Source: three-view drawing plus pictorial views. Frame: mm from the lowest corner of the part. A direction names the side the tool comes from. Give positions to 0.01 mm unless a question says otherwise; leave off trailing zeros. Write each loop counter-clockwise with the first axis right and the second up, starting at its lowest first coordinate (ties: lowest second). Pieces come first, ordered by that corner, then holes. Notation, with made-up numbers: M -14,-5.75 L 14,-5.75 A18 ccw 14,15.25 Z; hole C 57,82 d5. An arc over 180 degrees is marked long. Return JSON: item names as keys, results as strings.
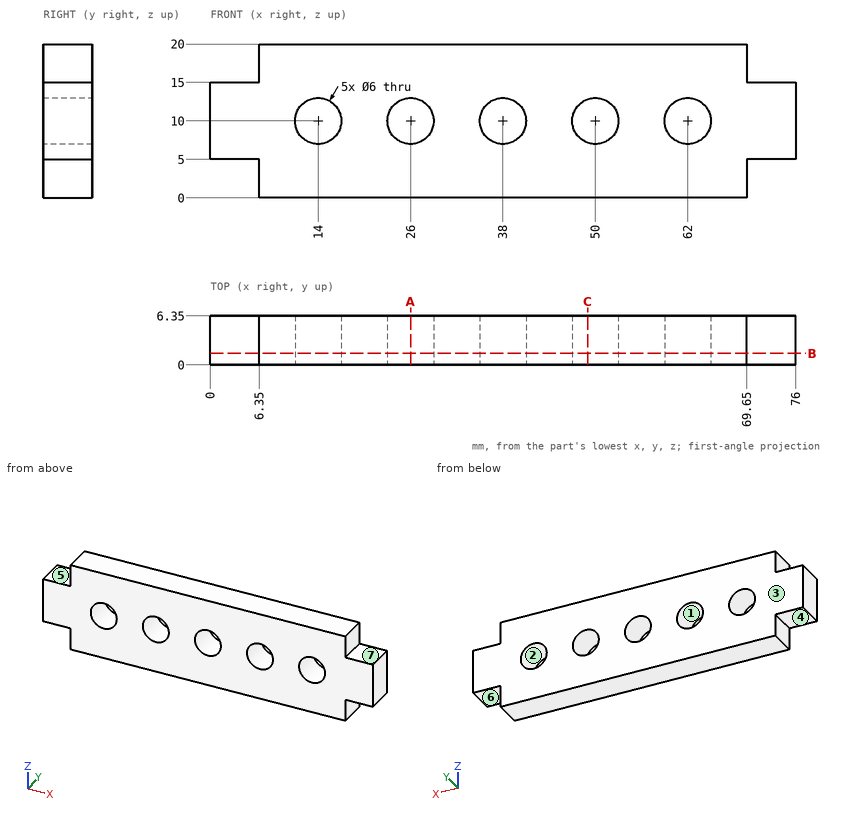
1) Line query: line 1 (X direction, y = 4, z = 10); line 2 (X direction, y = 3, z = 18); line 3 (Z direction, x = 51, y = 6). Output: solid intervals per line, ascending. Write a range as [from, to].
Numbers:
{"line 1": "x = [0, 11], [17, 23], [29, 35], [41, 47], [53, 59], [65, 76]", "line 2": "x = [6.35, 69.65]", "line 3": "z = [0, 7.17], [12.83, 20]"}
2) Cut plane A-A, the plane x = 26. Return the cut outline in (y, z), then the cut area to 3 significant figures.
Numbers:
{"outline": "M 0,0 L 6.35,0 L 6.35,7 L 0,7 Z; M 0,13 L 6.35,13 L 6.35,20 L 0,20 Z", "area": "88.9 mm²"}
3) Draft query along X for the marked faces 1, 2 and 3. Return one class per face: released by +X, released by -X, zero draft, split by the parting line, or undercut.
Numbers:
{"face 1": "undercut", "face 2": "undercut", "face 3": "zero draft"}
4) Contact query for flat-ended pins moving along their axis: pin 1 Ø3 at (x, y) = (73, 4.5) entering from +Z; pin 2 Ø2.5 at (y, z) = (2, 3) entering from +X. Output: stop coordinate, or through.
Numbers:
{"pin 1": "stops at z = 15", "pin 2": "stops at x = 69.65"}
5) Cut plane B-B, the plane y = 1.5. Return the cut outline in (x, z).
Numbers:
{"outline": "M 0,5 L 6.35,5 L 6.35,0 L 69.65,0 L 69.65,5 L 76,5 L 76,15 L 69.65,15 L 69.65,20 L 6.35,20 L 6.35,15 L 0,15 Z; hole C 14,10 d6; hole C 26,10 d6; hole C 38,10 d6; hole C 50,10 d6; hole C 62,10 d6"}
6) Cut plane C-C, the plane x = 49. Return the cut outline in (y, z), then the cut area to 3 significant figures.
Numbers:
{"outline": "M 0,0 L 6.35,0 L 6.35,7.17 L 0,7.17 Z; M 0,12.83 L 6.35,12.83 L 6.35,20 L 0,20 Z", "area": "91.1 mm²"}
7) Set-up query: the marked faces 4, 5, 6 and 7. Return all of +Z, -Z, +X, -X, +Y, -Y with unobstructed straight access to the full face (end or side cutting, diameter ignored); none if empty.
Numbers:
{"face 4": "-Z, -X, +Y, -Y", "face 5": "+Z, -X, +Y, -Y", "face 6": "-Z, +X, +Y, -Y", "face 7": "+Z, +X, +Y, -Y"}
